Read the model definition and answer for the solid it produces. Units are mm, in the model's axes. Face numbers are marked on the shaded views. Give positions to 0.01 mm unless a question says otherwise; leave off trailing zeros. Loops run counter-clockwise (first coordinate to the right, second up) from the corner with the lowest first, then second, coordinate; pieces in that order, holes last. Notation, with made-up numbers: (65, 10) -> (103, 10) arc R21 cw to (103, 46) -> close; hole circle Ø3 at (52.5, 87). An arc over 180 degrees is marked (long way). One line per item, written item: value. Start each with the question number.
from build123d import *

# Parameters (mm, degrees)
CYLINDER020_R     = 1.5
CYLINDER020_DEPTH = 22
TORUS003_R        = 0.9
TORUS002_R        = 0.9
CYLINDER018_R     = 11
CYLINDER018_DEPTH = 5
CYLINDER017_R     = 1.5
CYLINDER017_DEPTH = 10
CYLINDER019_R     = 2.5
CYLINDER019_DEPTH = 10


with BuildPart() as cylinder020:
    # Cylinder020 → Cylinder020 (new body)
    with BuildSketch(Plane.XY.offset(-4)):
        Circle(CYLINDER020_R)
    extrude(amount=CYLINDER020_DEPTH)


with BuildPart() as torus003:
    # Torus003 → Torus003 (revolve)
    with BuildSketch(Plane(origin=(0, 0, -0.5), x_dir=(1, 0, 0), z_dir=(0, -1, 0))):
        with Locations((10.8, 0)):
            Circle(TORUS003_R)
    revolve(axis=Axis((0, 0, -0.5), (0, 0, 1)))


with BuildPart() as torus002:
    # Torus002 → Torus002 (revolve)
    with BuildSketch(Plane(origin=(0, 0, 1.5), x_dir=(1, 0, 0), z_dir=(0, -1, 0))):
        with Locations((10.8, 0)):
            Circle(TORUS002_R)
    revolve(axis=Axis((0, 0, 1.5), (0, 0, 1)))


with BuildPart() as cylinder018:
    # Cylinder018 → Cylinder018 (new body)
    with BuildSketch(Plane.XY.offset(-2)):
        Circle(CYLINDER018_R)
    extrude(amount=CYLINDER018_DEPTH)


with BuildPart() as cylinder017:
    # Cylinder017 → Cylinder017 (new body)
    with BuildSketch(Plane.XY.offset(-2)):
        Circle(CYLINDER017_R)
    extrude(amount=CYLINDER017_DEPTH)


with BuildPart() as cut013:
    # Cylinder019 → Cylinder019 (new body)
    with BuildSketch(Plane.XY.offset(-2)):
        Circle(CYLINDER019_R)
    extrude(amount=CYLINDER019_DEPTH)

    # Cut010: cut Cylinder017
    add(cylinder017.part, mode=Mode.SUBTRACT)

    # Fusion012: union Cylinder018
    add(cylinder018.part)

    # Cut011: cut Torus002
    add(torus002.part, mode=Mode.SUBTRACT)

    # Cut012: cut Torus003
    add(torus003.part, mode=Mode.SUBTRACT)

    # Cut013: cut Cylinder020
    add(cylinder020.part, mode=Mode.SUBTRACT)


with BuildPart() as cut013_1:
    # Cut013 placement: moved
    add(cut013.part.moved(Location((47, 54, 16))))


solid = cut013_1.part
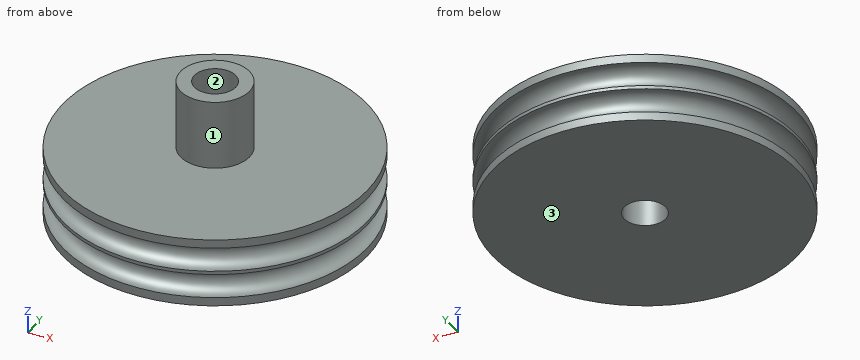
Item 1: Determine the mould class of the marked faces 1, 2 and 3 for opening direction Y: pulls with the +Y half, pulls with the -Y half, needs draft (parallel to the pull), parting line crosses it, or undercut.
Item 2: Section A-A, the plane y = 54 is taken. Determine the outline of the cut face in (x, z), plus the area to 3 significant figures.
Item 3: Section B-B, the plane x = 47 is taken. Determine the outline of the cut face in (y, z).
Item 4: Consider L1, parallel to Z at x = 54.5, y = 62; L2, parallel to Z at x = 47.25, y = 44; L3, parallel to Z at x = 38.25, y = 58.5. Determine where each line is inside the solid, lowest interval first. Write a range as [from, to].
Item 5: Section C-C, the plane z = 21.25 is taken. Determine the outline of the cut face in (x, y).
Item 6: Flat-ended cylindrical pins translate along their axes: pin 1 (4 mm diameter, centred on x = 46, z = 22.5, fed in from +Y); pin 2 (3.5 mm diameter, centred on x = 47, y = 54, fed in from +Z); pin 3 (6 mm diameter, centred on y = 60, z = 20, fed in from +X); pin 4 (2 mm diameter, centred on x = 41.5, z = 16.5, fed in from -Y). Find the tip coordinate at first contact, or state that the pin passes through.
Computed values:
1. face 1: parting line crosses it
1. face 2: undercut
1. face 3: needs draft
2. outline: (36, 14) -> (45.5, 14) -> (45.5, 24) -> (44.5, 24) -> (44.5, 19) -> (36, 19) -> (36, 18.38) arc R0.9 cw (long way) to (36, 16.62) -> (36, 16.38) arc R0.9 cw (long way) to (36, 14.62) -> close; (48.5, 14) -> (58, 14) -> (58, 14.62) arc R0.9 cw (long way) to (58, 16.38) -> (58, 16.62) arc R0.9 cw (long way) to (58, 18.38) -> (58, 19) -> (49.5, 19) -> (49.5, 24) -> (48.5, 24) -> close
2. area: 98.5 mm²
3. outline: (43, 14) -> (52.5, 14) -> (52.5, 24) -> (51.5, 24) -> (51.5, 19) -> (43, 19) -> (43, 18.38) arc R0.9 cw (long way) to (43, 16.62) -> (43, 16.38) arc R0.9 cw (long way) to (43, 14.62) -> close; (55.5, 14) -> (65, 14) -> (65, 14.62) arc R0.9 cw (long way) to (65, 16.38) -> (65, 16.62) arc R0.9 cw (long way) to (65, 18.38) -> (65, 19) -> (56.5, 19) -> (56.5, 24) -> (55.5, 24) -> close
4. L1: [14, 14.62], [16.38, 16.62], [18.38, 19]
4. L2: [14, 15.08], [15.92, 17.08], [17.92, 19]
4. L3: [14, 19]
5. outline: circle Ø5 at (47, 54); hole circle Ø3 at (47, 54)
6. pin 1: y = 56.5
6. pin 2: z = 24
6. pin 3: x = 57.53
6. pin 4: y = 43.96
